Check sheet for the modelled part. Datum: model origin and axes. Units: mm. A direction names the side the tool comes from. Round coordinates to 2 decimals unless told otherwise and drop trailing zeros. Order: outer loops, then holes, each group sorted by start corner. A loop starts at its lowest first (then second) coordinate and runs counter-clockwise, first axis right, second up.
(1) Thickness scan on probe 1 along Y at (x, z) = (17.5, 16.5); probe 2 along Z at (x, y) = (-7.5, 36); probe 3 along X at (y, z) = (33, 48.5). Record the ranges inside material, lowest first.
(2) Sectioned sample at D-D, the plane y = 24.5. Enter the section's corners in (x, z).
(3) Depth check by flat-ended pin: pin 1 (1.5 mm diameter, centred on y = 4.5, z = 15, fed in from -X); pin 2 (3 mm diameter, centred on y = 28.5, z = 31.5, fed in from +X); pin 3 (11.5 mm diameter, centred on x = -4, z = 32, fed in from -Y). Enter the tip coordinate at first touch or a pass-through.
(4) Sectioned sample at A-A, the plane y = 16. Enter the section's corners in (x, z), and give its area (3 significant figures).
(5) Tool access check on faces 1 (the flat face through (16, 13, 25.4)), 2 (the flat face through (12.7, 26, 36)), 3 (the cylindrical face through (1.449, 5.724, 23.872)), 4 (the cylindrical face through (12.807, 1.528, 23.951)), 5 (the flat face through (-10, 26, 12.7)). Record the directions out of +Z, -Z, +X, -X, +Y, -Y that give a thin tool (end or side, any length) a straight path to the whole face; none if there is none.
(6) Sectioned sample at B-B, the plane z = 9. Enter the section's corners in (x, y).
```python
from build123d import *

# Parameters (mm, degrees)
F0_W     = 25.4
F0_H     = 25.4
F1_DEPTH = 25.4
F2_R     = 5.08
F3_W     = 7.62
F3_H     = 7.62
F4_DEPTH = 19.05


with BuildPart() as f1:
    # F0 (on Front) → F1 (new body)
    with BuildSketch(Plane.XZ):
        with Locations((12.7, 12.7)):
            Rectangle(F0_W, F0_H)
    extrude(amount=-F1_DEPTH)

    # F2
    f2_edges = [f1.edges().sort_by_distance(p)[0] for p in [
        (25.4, 12.7, 25.4),
        (0, 12.7, 25.4),
        (12.7, 0, 25.4),
        (12.7, 25.4, 25.4),
        (0, 0, 12.7),
        (12.7, 0, 0),
        (25.4, 0, 12.7),
        (25.4, 12.7, 0),
        (25.4, 25.4, 12.7),
        (0, 12.7, 0),
        (0, 25.4, 12.7),
        (12.7, 25.4, 0),
    ]]
    fillet(f2_edges, radius=F2_R)

    # F3 (on face) → F4 (join, symmetric)
    with BuildSketch(Plane(origin=(0, 25.4, 0), x_dir=(-1, 0, 0), z_dir=(0, 1, 0))):
        with Locations((-8.89, 16.51)):
            Rectangle(F3_W, F3_H)
        Polygon((-5.08, 20.32), (-5.08, 12.7), (25.4, 12.7), (25.4, 50.8), (-12.7, 50.8), (-12.7, 20.32), align=None)
    extrude(amount=F4_DEPTH, both=True)


solid = f1.part
```
Derived:
1. probe 1: y = 0 to 25.4
1. probe 2: z = 12.7 to 50.8
1. probe 3: x = -25.4 to 12.7
2. outline: (-25.4, 12.7) - (2.19, 12.7) - (2.19, 5.08) arc R2.89 ccw to (5.08, 2.19) - (20.32, 2.19) arc R2.89 ccw to (23.21, 5.08) - (23.21, 20.32) arc R2.89 ccw to (20.32, 23.21) - (12.7, 23.21) - (12.7, 50.8) - (-25.4, 50.8) - close
3. pin 1: stops at x = 0
3. pin 2: stops at x = 12.7
3. pin 3: stops at y = 6.35
4. outline: (-25.4, 12.7) - (0, 12.7) - (0, 5.08) arc R5.08 ccw to (5.08, 0) - (20.32, 0) arc R5.08 ccw to (25.4, 5.08) - (25.4, 20.32) arc R5.08 ccw to (20.32, 25.4) - (12.7, 25.4) - (12.7, 50.8) - (-25.4, 50.8) - close
4. area: 1,920 mm2
5. face 1: +Z, +X, -Y
5. face 2: +Z, +X, +Y
5. face 3: +Z, -X, -Y
5. face 4: +Z, +X, -X, -Y
5. face 5: -Z, -X, +Y
6. outline: (0, 5.08) arc R5.08 ccw to (5.08, 0) - (20.32, 0) arc R5.08 ccw to (25.4, 5.08) - (25.4, 20.32) arc R5.08 ccw to (20.32, 25.4) - (5.08, 25.4) arc R5.08 ccw to (0, 20.32) - close
